Work out the finished part from the listing and answer in its coordinate system (mm). Face numbers are marked on the shaded views. A direction names the side the tool comes from. Round coordinates to 2 decimals unless told otherwise and drop trailing zeros. Loops run counter-clockwise (first coordinate to the right, second up) from the corner with the lowest first, then second, coordinate; pieces in that order, holes last. Notation, with made-up numbers: M 39.5,46 L 58.5,46 A25 ccw 58.5,79 Z; hole C -10,-33.75 d9. An arc over 180 degrees is marked long. One line per item, written item: value.
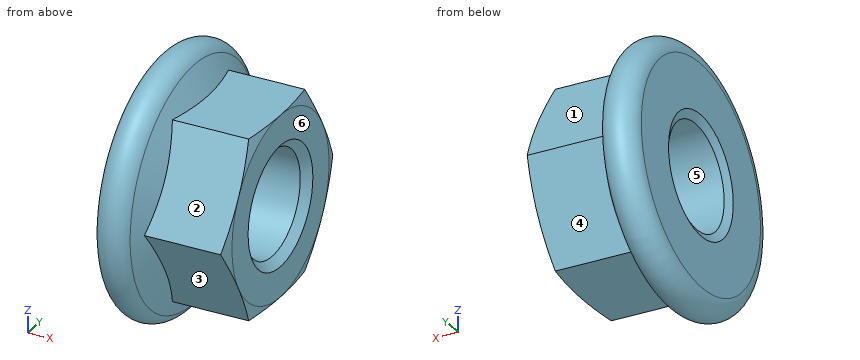
Autodesk Inventor part; units mm, degrees
ref_plane "Work Plane1" through (63.747, 0, 0) normal (0, 0, -1) x (-1, 0, 0)
ref_plane "YZ Plane" through (0, 0, 0) normal (1, 0, 0) x (0, 1, 0)
ref_plane "XZ Plane" through (0, 0, 0) normal (0, 1, 0) x (-1, 0, 0)
sketch "Эскиз1" plane through (0, 0, 0) normal (0, 0, 1) x (1, 0, 0)
  line L0 (-4.6105, 0) -> (24.1018, 0)
  line L1 (7.8956, 15) -> (5.7189, 19.6679)
  line L2 (7.8956, 15) -> (20, 15) construction
  line L3 (20, 15) -> (20, 0) construction
  arc A0 (5.7189, 19.6679) -> (0, 18.4) centre (3, 18.4) ccw
  line L4 (7.8956, 15) -> (7.8956, 0)
  line L5 (0, -4.3926) -> (0, 26.3554)
  point P0 (0, 0)
  dimension "d2" = 30
  dimension "d4" = 42.8
  dimension "d5" = 3
  dimension "d15" = 20
  dimension "d16" = 25
revolve "Кольцо" add sketch "Эскиз1" angle 360 about axis through (-10, 0, 0) along (1, 0, 0)
sketch "Эскиз2" plane through (0, 0, 0) normal (-1, 0, 0) x (0, 0, 1)
  circle A0 centre (0, 0) radius 4.9
  line L0 (-15, -8.6603) -> (-15, 8.6603)
  line L1 (-15, 8.6603) -> (0, 17.3205)
  line L2 (0, 17.3205) -> (15, 8.6603)
  line L3 (15, 8.6603) -> (15, -8.6603)
  line L4 (15, -8.6603) -> (0, -17.3205)
  line L5 (0, -17.3205) -> (-15, -8.6603)
  circle A1 centre (0, 0) radius 18.4
  dimension "d6" = 34.641
extrude "Базовый элемент" add sketch "Эскиз2" against normal blind 20 contours A0 | L0 L1 L2 L3 L4 L5
sketch "Эскиз3" plane through (0, 0, 0) normal (0, 0, 1) x (1, 0, 0)
  line L0 (6.8135, 17.3205) -> (20, 17.3205)
  line L1 (20, 8.6603) -> (20, 17.3205)
  line L2 (0, -18.4) -> (0, 18.4)
  line L3 (-4, 0) -> (24, 0)
  line L4 (19.3782, 17.3205) -> (20, 15)
  dimension "d10" = 15
  dimension "d11" = 30
revolve "Фаска1" cut sketch "Эскиз3" angle 360 about axis through (-10, 0, 0) along (1, 0, 0)
sketch "Эскиз4" plane through (0, 0, 0) normal (-1, 0, 0) x (0, 0, 1)
  circle A0 centre (0, 0) radius 18.4
hole "Резьба" at (0, 0, 0) direction (1, 0, 0) diameter 17.294 end through all
chamfer "Фаска2" distance 1.3532 angle 30 1 edges at (0, 0, -8.647) measured on face at (0, 14.9498, -1.8152)
ref_plane "Work Plane1" through (63.747, 0, 0) normal (0, 0, -1) x (-1, 0, 0)
chamfer "Фаска3" distance 1.3532 angle 45 1 edges at (20, 0, -8.647)
equation "\"d6\" = 1.1547 * SW"
equation "\"d7\" = KOH"
equation "\"d12\" = -0.5 * GD1 + 0.5 * NND"
equation "\"d46\" = -0.5 * GD1 + 0.5 * NND"
equation "\"d51\" = -0.5 * GD1 + 0.5 * NND"
equation "\"d2\" = SW"
equation "\"d4\" = LADI"
equation "\"d5\" = PHH"
equation "\"d15\" = KOH"
equation "\"d16\" = KEWI"
equation "\"d10\" = ANG1"
equation "\"d11\" = SW0"
equation "\"ANG1\" = 15deg"
equation "\"KEWI\" = 25deg"
equation "\"LADI\" = 42.8"
equation "\"SW\" = 30"
equation "\"PHH\" = RR"
equation "\"KOH\" = NND"
equation "\"SW0\" = SW"
equation "\"d1\" = LADI"
equation "\"d3\" = PHH"
equation "\"GUL\" = 0.541266 * PTC"
equation "\"RR\" = 3"
equation "\"TOA\" = 30deg"
equation "\"PTC\" = 2.5"
equation "\"GAL\" = 0.541266 * PTC"
equation "\"E0\" = 1.155 * SW"
properties part number "DIN 6923 - M20" material "Сталь, мягкая"
1) Each of these flat-tipped pins is pushed along its axis until it touches: pin 1 (8 mm diameter, centred on x = 13.5, z = 0.5, fed in from -Y); pin 2 (1.5 mm diameter, centred on x = 3, y = -15, fed in from +Z); pin 3 (6 mm diameter, centred on x = 14, y = 9, fed in from -Z). Where does it stop, or does it pass through?
Check values:
pin 1: y = -17.32
pin 2: z = 15.97
pin 3: z = -15
2) Find section A-A (x = 12). Give the vertices of the cut face in (y, z), then the cut area to 3 significant figures.
Check values:
outline: M -17.32,0 L -8.66,-15 L 8.66,-15 L 17.32,0 L 8.66,15 L -8.66,15 Z; hole C 0,0 d17.29
area: 545 mm2
3) The mould has two halves that part along Y. Classify the marked faces 4, 5 and 6: +Y half, -Y half, draft (parallel to the pull), parting line (faces both ways), or undercut.
Check values:
face 4: +Y half
face 5: undercut
face 6: draft
4) Find the intervals of material crossed by probe 1 along Y at (x, z) = (12.5, 0); probe 2 along Z at (x, y) = (10.75, 0); probe 3 along Y at (x, z) = (11, 7), in increasing order. Write a range as from..to.
Check values:
probe 1: -17.32..-8.65, 8.65..17.32
probe 2: -15..-8.65, 8.65..15
probe 3: -13.28..-5.08, 5.08..13.28
5) For the marked faces 1, 2 and 3, determine the directions among +Z, -Z, +X, -X, +Y, -Y from which every point of the face is accessible in a straight line to the end or side of a thin tool.
Check values:
face 1: +Z, +X, +Y
face 2: +Z, +X, -Y
face 3: -Z, +X, -Y
